Build history of the part. All positions in model axes, mm. A direction names the side the tool comes from. Round coordinates to 2 decimals unless told otherwise and drop trailing zeros. Loops run counter-clockwise (first coordinate to the right, second up) from the corner with the lowest first, then second, coordinate; pieces in that order, holes last. Notation, with made-up numbers: (38, -14) - (52, -14) arc R17 cw to (52, -3) - close; hole circle Ø3 at (14, 89). An arc over 180 degrees is marked (long way). Use a Markdown table: item, result.
Autodesk Inventor part; units mm, degrees
ref_plane "YZ Plane" through (0, 0, 0) normal (1, 0, 0) x (0, 1, 0)
ref_plane "XZ Plane" through (0, 0, 0) normal (0, 1, 0) x (-1, 0, 0)
ref_plane "XY Plane" through (0, 0, 0) normal (0, 0, 1) x (1, 0, 0)
sketch "Sketch1" plane through (0, 0, 0) normal (0, 0, 1) x (1, 0, 0)
  line L0 (19.9924, -21.8579) -> (16.7724, -25.0779)
  line L1 (19.9924, -21.8579) -> (19.9924, 20.4221)
  arc A0 (19.9924, 20.4221) -> (14.4924, 25.9221) centre (14.4924, 20.4221) ccw construction
  line L2 (14.4924, 25.9221) -> (14.2174, 25.9221)
  line L3 (14.2174, 25.9221) -> (14.2174, 26.4221)
  line L4 (9.7174, 30.9221) -> (14.2174, 26.4221)
  line L5 (-3.2826, 30.9221) -> (3.2174, 30.9221)
  line L6 (-7.7826, 26.4221) -> (-3.2826, 30.9221)
  line L7 (-7.7826, 25.9221) -> (-7.7826, 26.4221)
  line L8 (-7.7826, 25.9221) -> (-16.5076, 25.9221)
  arc A1 (-16.5076, 25.9221) -> (-22.0076, 20.4221) centre (-16.5076, 20.4221) ccw construction
  line L9 (-22.0076, 20.4221) -> (-22.0076, -10.5779)
  arc A2 (-22.0076, -10.5779) -> (-16.5076, -16.0779) centre (-16.5076, -10.5779) ccw construction
  line L10 (-16.5076, -16.0779) -> (-13.0076, -16.0779)
  line L11 (-13.0076, -16.0779) -> (-13.0076, -21.8579)
  line L12 (-9.7876, -25.0779) -> (-13.0076, -21.8579)
  line L13 (-9.7876, -25.0779) -> (-9.7826, -25.0779)
  line L14 (-12.7826, -28.0779) -> (-9.7826, -25.0779)
  line L15 (-15.5326, -28.0779) -> (-12.7826, -28.0779)
  line L16 (-15.5326, -28.0779) -> (-15.5326, -66.0779)
  arc A3 (-15.5326, -66.0779) -> (-9.5326, -72.0779) centre (-9.5326, -66.0779) ccw
  line L17 (-9.5326, -72.0779) -> (15.9674, -72.0779)
  arc A4 (15.9674, -72.0779) -> (21.9674, -66.0779) centre (15.9674, -66.0779) ccw
  line L18 (21.9674, -28.0779) -> (21.9674, -66.0779)
  line L19 (19.2174, -28.0779) -> (21.9674, -28.0779)
  line L20 (19.2174, -28.0779) -> (16.2174, -25.0779)
  line L21 (16.2174, -25.0779) -> (16.7724, -25.0779)
  circle A5 centre (-16.5076, 20.4221) radius 1.7 construction
  circle A6 centre (14.4924, 20.4221) radius 1.7 construction
  circle A7 centre (14.4924, -10.5779) radius 1.7 construction
  circle A8 centre (-16.5076, -10.5779) radius 1.7 construction
  circle A9 centre (14.7174, -41.5779) radius 2.25
  circle A10 centre (-8.2826, -41.5779) radius 2.25
  circle A11 centre (14.7174, -64.5779) radius 2.25
  circle A12 centre (-8.2826, -64.5779) radius 2.25
  circle A13 centre (-1.0076, 4.9221) radius 12.5 construction
  line L22 (-20.0076, 25.9221) -> (17.9924, 25.9221)
  line L23 (19.9924, 23.9221) -> (19.9924, -14.0779)
  line L24 (17.9924, -16.0779) -> (-20.0076, -16.0779)
  line L25 (-22.0076, -14.0779) -> (-22.0076, 23.9221)
  line L26 (-22.0076, 25.9221) -> (19.9924, -16.0779) construction
  line L27 (19.9924, 25.9221) -> (-22.0076, -16.0779) construction
  line L28 (-20.0076, 25.9221) -> (-22.0076, 23.9221)
  line L29 (17.9924, 25.9221) -> (19.9924, 23.9221)
  line L30 (19.9924, -14.0779) -> (17.9924, -16.0779)
  line L31 (-20.0076, -16.0779) -> (-22.0076, -14.0779)
  line L32 (7.7174, 40.9221) -> (8.8956, 39.0987)
  line L33 (5.2174, 40.9221) -> (7.7174, 40.9221)
  line L34 (3.2174, 38.9221) -> (5.2174, 40.9221)
  line L35 (3.2174, 30.9221) -> (3.2174, 38.9221)
  arc A14 (8.8956, 39.0987) -> (9.7174, 30.9221) centre (18.3776, 35.9221) ccw
  point P0 (0, 0)
  dimension "d0" = 2
  dimension "d1" = 2
  dimension "d2" = 2
  dimension "d3" = 2
  dimension "d4" = 2
  dimension "d5" = 2
  dimension "d6" = 2
  dimension "d7" = 2
extrude "Extrusion1" add sketch "Sketch1" along normal blind 31 contours L30 L24 L10 L31 L25 L9 L28 L22 L8 L2 L29 L23 L1
sketch "Sketch2" plane through (0, 0, 0) normal (0, 0, -1) x (-1, 0, 0)
  circle A0 centre (1.0076, 4.9221) radius 12.5
  circle A1 centre (1.0076, 4.9221) radius 11
  point P0 (0, 0)
  dimension "d10" = 22
extrude "Extrusion2" add sketch "Sketch2" along normal blind 2 contours A1
sketch "Sketch3" plane through (0, 0, 0) normal (0, 0, -1) x (-1, 0, 0)
  line L0 (20.0076, 25.9221) -> (22.0076, 23.9221)
  line L1 (-19.9924, 23.9221) -> (-17.9924, 25.9221)
  line L2 (-17.9924, -16.0779) -> (-19.9924, -14.0779)
  line L3 (22.0076, -14.0779) -> (20.0076, -16.0779)
  circle A0 centre (-14.4924, 20.4221) radius 1.5
  circle A1 centre (16.5076, 20.4221) radius 1.5
  line L4 (-18.9924, 24.9221) -> (21.0076, -15.0779) construction
  line L5 (21.0076, 24.9221) -> (-18.9924, -15.0779) construction
  circle A2 centre (-14.4924, -10.5779) radius 1.5
  circle A3 centre (16.5076, -10.5779) radius 1.5
  point P0 (0, 0)
  dimension "d13" = 31
  dimension "d14" = 3
extrude "Extrusion3" cut sketch "Sketch3" against normal blind 5
sketch "Sketch4" plane through (-1.0076, 4.9221, -2) normal (0, 0, -1) x (-1, 0, 0)
  circle A0 centre (0, 0) radius 11
  circle A1 centre (0, 0) radius 2.5
  point P0 (-1.0076, -4.9221)
  dimension "d17" = 5
extrude "Extrusion4" add sketch "Sketch4" along normal blind 24 contours A1
equation "\"d1\" = d0"
equation "\"d2\" = d0"
equation "\"d3\" = d2"
equation "\"d4\" = d0"
equation "\"d5\" = d4"
equation "\"d6\" = d0"
equation "\"d7\" = d6"
properties part number "NEMA17"
Q1. Cut at A-A, the plane x = 0. List the corners of the cut face in (y, z), plus the area to 3 significant figures.
Results found:
| item | result |
|---|---|
| outline | (-16.08, 0) - (-6.03, 0) - (-6.03, -2) - (2.63, -2) - (2.63, -26) - (7.21, -26) - (7.21, -2) - (15.88, -2) - (15.88, 0) - (25.92, 0) - (25.92, 31) - (-16.08, 31) - close |
| area | 1,460 mm2 |
Q2. Which spindle directions (+Z, -Z, +X, -X, +Y, -Y) get a long thin tool onto all of the face, cutting with end or side? Do faces 1 (the face through (-16, 20, 5)), 2 (the face through (-20.99, 24.94, 15.28)). Say none if no direction does.
Results found:
| item | result |
|---|---|
| face 1 | -Z |
| face 2 | +Z, -Z, -X, +Y |
Q3. Cut at D-D, the plane z = -13.5. List the corners of the cut face in (x, y), plus the area to 3 significant figures.
Results found:
| item | result |
|---|---|
| outline | circle Ø5 at (-1.01, 4.92) |
| area | 19.6 mm2 |
Q4. Drop flat-ended pins along their axis: pin 1 (2.5 mm diameter, centred on x = -16.5, y = 20.5, fed in from -Z); pin 2 (3.5 mm diameter, centred on x = -16.51, y = -10.58, fed in from -Z); pin 3 (6.5 mm diameter, centred on x = -6, y = 8.5, fed in from -Z). Give the stop position or say it passes through.
Results found:
| item | result |
|---|---|
| pin 1 | stops at z = 5 |
| pin 2 | stops at z = 0 |
| pin 3 | stops at z = -2 |
Q5. Cut at B-B, the plane y = -3.5. List the corners of the cut face in (x, z).
Results found:
| item | result |
|---|---|
| outline | (-22.01, 0) - (-8.08, 0) - (-8.08, -2) - (6.07, -2) - (6.07, 0) - (19.99, 0) - (19.99, 31) - (-22.01, 31) - close |
Q6. Probe line 1 (Y direction, x = 14.5, z = 1); line 2 (Z direction, x = 8.5, y = 11.5); line 3 (Z direction, x = -5.5, y = -1.5). List the from-to ranges inside material, lowest first.
Results found:
| item | result |
|---|---|
| line 1 | y = -16.08 to -12.08, -9.08 to 18.92, 21.92 to 25.92 |
| line 2 | z = 0 to 31 |
| line 3 | z = -2 to 31 |
Q7. Cut at C-C, the plane x = -6.5. List the corners of the cut face in (y, z), plus the area to 3 significant figures.
Results found:
| item | result |
|---|---|
| outline | (-16.08, 0) - (-4.61, 0) - (-4.61, -2) - (14.45, -2) - (14.45, 0) - (25.92, 0) - (25.92, 31) - (-16.08, 31) - close |
| area | 1,340 mm2 |
